Input: part model. Units: mm. Frame: model coordinates. Face numbers are marked on the shaded views. A direction names the side the tool comes from. Give positions to 0.01 mm unless a question says otherwise; leave off trailing zeros. Write each loop counter-clockwise with the first axis right and the second up, starting at its lowest first coordinate (ties: lowest second). Pieces come first, ordered by that corner, then holes. Notation, with made-up numbers: (53.25, 43.5) - (73.25, 43.5) arc R21 ccw to (73.25, 55.5) - close; hole circle Ø10 at (48, 78). An arc over 180 degrees is marked (long way). Answer as CSV lines item,"result".
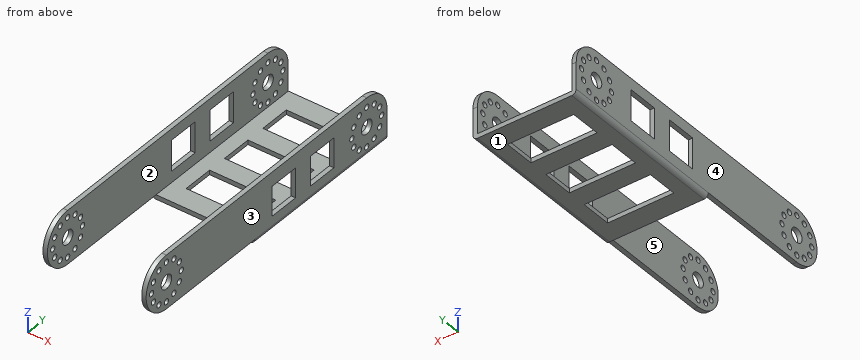
```python
from build123d import *

# Parameters (mm, degrees)
ESQUISSE2_W        = 33.6
ESQUISSE2_H        = 62
ESQUISSE2_W_2      = 23.6
ESQUISSE2_H_2      = 11
BOSS_EXTRU_1_DEPTH = 1.5875
ESQUISSE3_R        = 2.5
ESQUISSE3_R_2      = 1
ESQUISSE3_W        = 10.5875
ESQUISSE3_H        = 11
BOSS_EXTRU_2_DEPTH = 1.5875
CONG_3_R           = 1.5875
CONG_4_R           = 9.5
ESQUISSE4_R        = 2.5
ESQUISSE4_R_2      = 1
ESQUISSE4_W        = 11.003569346
ESQUISSE4_H        = 11
BOSS_EXTRU_3_DEPTH = 1.5875
CONG_6_R           = 1.5875
CONG_7_R           = 9.5


with BuildPart() as part:
    # Esquisse2 → Boss.-Extru.1 (new body)
    with BuildSketch(Plane.XY):
        Rectangle(ESQUISSE2_W, ESQUISSE2_H)
        Rectangle(ESQUISSE2_W_2, ESQUISSE2_H_2, mode=Mode.SUBTRACT)
        with Locations((0, 18)):
            Rectangle(ESQUISSE2_W_2, ESQUISSE2_H_2, mode=Mode.SUBTRACT)
        with Locations((0, -18)):
            Rectangle(ESQUISSE2_W_2, ESQUISSE2_H_2, mode=Mode.SUBTRACT)
    extrude(amount=BOSS_EXTRU_1_DEPTH)


with BuildPart() as body_2:
    # Esquisse3 → Boss.-Extru.2 (new body)
    with BuildSketch(Plane(origin=(16.8, 0, 0), x_dir=(0, 0, -1), z_dir=(1, 0, 0))):
        with BuildLine():
            Line((-20.5875, 31), (0, 31))
            Line((0, 31), (0, -31))
            Line((0, -31), (-1.5875, -31))
            Line((-1.5875, -31), (-1.5875, -72.5))
            ThreePointArc((-1.5875, -72.5), (-11.0875, -82), (-20.5875, -72.5))
            Line((-20.5875, -72.5), (-20.5875, -31))
            Line((-20.5875, -31), (-20.5875, 31))
        make_face()
        with Locations((-11.0875, -72.5)):
            Circle(ESQUISSE3_R, mode=Mode.SUBTRACT)
        with Locations((-11.0875, -79.5)):
            Circle(ESQUISSE3_R_2, mode=Mode.SUBTRACT)
        with Locations((-14.5875, -78.562177826)):
            Circle(ESQUISSE3_R_2, mode=Mode.SUBTRACT)
        with Locations((-17.149677826, -76)):
            Circle(ESQUISSE3_R_2, mode=Mode.SUBTRACT)
        with Locations((-18.0875, -72.5)):
            Circle(ESQUISSE3_R_2, mode=Mode.SUBTRACT)
        with Locations((-17.149677826, -69)):
            Circle(ESQUISSE3_R_2, mode=Mode.SUBTRACT)
        with Locations((-14.5875, -66.437822174)):
            Circle(ESQUISSE3_R_2, mode=Mode.SUBTRACT)
        with Locations((-11.0875, -65.5)):
            Circle(ESQUISSE3_R_2, mode=Mode.SUBTRACT)
        with Locations((-7.5875, -66.437822174)):
            Circle(ESQUISSE3_R_2, mode=Mode.SUBTRACT)
        with Locations((-5.025322174, -69)):
            Circle(ESQUISSE3_R_2, mode=Mode.SUBTRACT)
        with Locations((-4.0875, -72.5)):
            Circle(ESQUISSE3_R_2, mode=Mode.SUBTRACT)
        with Locations((-5.025322174, -76)):
            Circle(ESQUISSE3_R_2, mode=Mode.SUBTRACT)
        with Locations((-7.5875, -78.562177826)):
            Circle(ESQUISSE3_R_2, mode=Mode.SUBTRACT)
        with Locations((-10.29375, 21.5)):
            Circle(ESQUISSE3_R, mode=Mode.SUBTRACT)
        with Locations((-10.29375, 28.5)):
            Circle(ESQUISSE3_R_2, mode=Mode.SUBTRACT)
        with Locations((-6.79375, 27.562177826)):
            Circle(ESQUISSE3_R_2, mode=Mode.SUBTRACT)
        with Locations((-4.231572174, 25)):
            Circle(ESQUISSE3_R_2, mode=Mode.SUBTRACT)
        with Locations((-3.29375, 21.5)):
            Circle(ESQUISSE3_R_2, mode=Mode.SUBTRACT)
        with Locations((-4.231572174, 18)):
            Circle(ESQUISSE3_R_2, mode=Mode.SUBTRACT)
        with Locations((-6.79375, 15.437822174)):
            Circle(ESQUISSE3_R_2, mode=Mode.SUBTRACT)
        with Locations((-10.29375, 14.5)):
            Circle(ESQUISSE3_R_2, mode=Mode.SUBTRACT)
        with Locations((-13.79375, 15.437822174)):
            Circle(ESQUISSE3_R_2, mode=Mode.SUBTRACT)
        with Locations((-16.355927826, 18)):
            Circle(ESQUISSE3_R_2, mode=Mode.SUBTRACT)
        with Locations((-17.29375, 21.5)):
            Circle(ESQUISSE3_R_2, mode=Mode.SUBTRACT)
        with Locations((-16.355927826, 25)):
            Circle(ESQUISSE3_R_2, mode=Mode.SUBTRACT)
        with Locations((-13.79375, 27.562177826)):
            Circle(ESQUISSE3_R_2, mode=Mode.SUBTRACT)
        with Locations((-10.29375, 0.597470968)):
            Rectangle(ESQUISSE3_W, ESQUISSE3_H, mode=Mode.SUBTRACT)
        with Locations((-10.29375, -17.402529032)):
            Rectangle(ESQUISSE3_W, ESQUISSE3_H, mode=Mode.SUBTRACT)
    extrude(amount=BOSS_EXTRU_2_DEPTH)

    # Congé3
    cong_3_edges = [body_2.edges().sort_by_distance(p)[0] for p in [
        (18.3875, 0, 0),
    ]]
    fillet(cong_3_edges, radius=CONG_3_R - 0.0001)  # a hair under: the kernel refuses the full size

    # Congé4
    cong_4_edges = [body_2.edges().sort_by_distance(p)[0] for p in [
        (17.59375, 31, 20.5875),
    ]]
    fillet(cong_4_edges, radius=CONG_4_R)

    # Intersect1: read off the stored shape, not the designer's step
    # Intersect1: union part
    add(part.part)

    # Esquisse4 → Boss.-Extru.3 (add)
    with BuildSketch(Plane.ZY.offset(16.8)):
        with BuildLine():
            Line((1.5875, 31), (0, 31))
            Line((0, 31), (0, -31))
            Line((0, -31), (1.5875, -31))
            Line((1.5875, -31), (1.5875, -72.5))
            ThreePointArc((1.5875, -72.5), (11.0875, -82), (20.5875, -72.5))
            Line((20.5875, -72.5), (20.5875, 31))
            Line((20.5875, 31), (1.5875, 31))
        make_face()
        with Locations(Location((11.0875, -72.5, 0), (0, 0, 180))):
            Circle(ESQUISSE4_R, mode=Mode.SUBTRACT)
        with Locations(Location((11.0875, -79.5, 0), (0, 0, 180))):
            Circle(ESQUISSE4_R_2, mode=Mode.SUBTRACT)
        with Locations(Location((7.5875, -78.562177826, 0), (0, 0, 180))):
            Circle(ESQUISSE4_R_2, mode=Mode.SUBTRACT)
        with Locations(Location((5.025322174, -76, 0), (0, 0, 180))):
            Circle(ESQUISSE4_R_2, mode=Mode.SUBTRACT)
        with Locations(Location((4.0875, -72.5, 0), (0, 0, 180))):
            Circle(ESQUISSE4_R_2, mode=Mode.SUBTRACT)
        with Locations(Location((5.025322174, -69, 0), (0, 0, 180))):
            Circle(ESQUISSE4_R_2, mode=Mode.SUBTRACT)
        with Locations(Location((7.5875, -66.437822174, 0), (0, 0, 180))):
            Circle(ESQUISSE4_R_2, mode=Mode.SUBTRACT)
        with Locations(Location((11.0875, -65.5, 0), (0, 0, 180))):
            Circle(ESQUISSE4_R_2, mode=Mode.SUBTRACT)
        with Locations(Location((14.5875, -66.437822174, 0), (0, 0, 180))):
            Circle(ESQUISSE4_R_2, mode=Mode.SUBTRACT)
        with Locations(Location((17.149677826, -69, 0), (0, 0, 180))):
            Circle(ESQUISSE4_R_2, mode=Mode.SUBTRACT)
        with Locations(Location((18.0875, -72.5, 0), (0, 0, 180))):
            Circle(ESQUISSE4_R_2, mode=Mode.SUBTRACT)
        with Locations(Location((17.149677826, -76, 0), (0, 0, 180))):
            Circle(ESQUISSE4_R_2, mode=Mode.SUBTRACT)
        with Locations(Location((14.5875, -78.562177826, 0), (0, 0, 180))):
            Circle(ESQUISSE4_R_2, mode=Mode.SUBTRACT)
        with Locations(Location((10.29375, 21.5, 0), (0, 0, 180))):
            Circle(ESQUISSE4_R, mode=Mode.SUBTRACT)
        with Locations(Location((6.79375, 15.437822174, 0), (0, 0, 180))):
            Circle(ESQUISSE4_R_2, mode=Mode.SUBTRACT)
        with Locations(Location((4.231572174, 18, 0), (0, 0, 180))):
            Circle(ESQUISSE4_R_2, mode=Mode.SUBTRACT)
        with Locations(Location((10.29375, 14.5, 0), (0, 0, 180))):
            Circle(ESQUISSE4_R_2, mode=Mode.SUBTRACT)
        with Locations(Location((3.29375, 21.5, 0), (0, 0, 180))):
            Circle(ESQUISSE4_R_2, mode=Mode.SUBTRACT)
        with Locations(Location((4.231572174, 25, 0), (0, 0, 180))):
            Circle(ESQUISSE4_R_2, mode=Mode.SUBTRACT)
        with Locations(Location((6.79375, 27.562177826, 0), (0, 0, 180))):
            Circle(ESQUISSE4_R_2, mode=Mode.SUBTRACT)
        with Locations(Location((10.29375, 28.5, 0), (0, 0, 180))):
            Circle(ESQUISSE4_R_2, mode=Mode.SUBTRACT)
        with Locations(Location((13.79375, 27.562177826, 0), (0, 0, 180))):
            Circle(ESQUISSE4_R_2, mode=Mode.SUBTRACT)
        with Locations(Location((16.355927826, 25, 0), (0, 0, 180))):
            Circle(ESQUISSE4_R_2, mode=Mode.SUBTRACT)
        with Locations(Location((17.29375, 21.5, 0), (0, 0, 180))):
            Circle(ESQUISSE4_R_2, mode=Mode.SUBTRACT)
        with Locations(Location((16.355927826, 18, 0), (0, 0, 180))):
            Circle(ESQUISSE4_R_2, mode=Mode.SUBTRACT)
        with Locations(Location((13.79375, 15.437822174, 0), (0, 0, 180))):
            Circle(ESQUISSE4_R_2, mode=Mode.SUBTRACT)
        with Locations((11.085715327, -0.168943848)):
            Rectangle(ESQUISSE4_W, ESQUISSE4_H, mode=Mode.SUBTRACT)
        with Locations((11.085715327, -18.168943848)):
            Rectangle(ESQUISSE4_W, ESQUISSE4_H, mode=Mode.SUBTRACT)
    extrude(amount=BOSS_EXTRU_3_DEPTH)

    # Congé6
    cong_6_edges = [body_2.edges().sort_by_distance(p)[0] for p in [
        (-18.3875, 0, 0),
    ]]
    fillet(cong_6_edges, radius=CONG_6_R)

    # Congé7
    cong_7_edges = [body_2.edges().sort_by_distance(p)[0] for p in [
        (-17.59375, 31, 20.5875),
    ]]
    fillet(cong_7_edges, radius=CONG_7_R)


solid = body_2.part
```
Item 1: Reachability of the marked faces 1 and 2 from +Z, -Z, +X, -X, +Y, -Y: full face, straight path, thin tool, end or side. Return the list, or none.
The answers:
face 1,"-Z, +X, -X, +Y, -Y"
face 2,"+Z, +Y, -Y"
Item 2: Cut plane C-C on y = 0. Return the cut outline in (x, z) (1 decimal).
The answers:
outline,"(-18.4, 1.6) arc R1.6 ccw to (-16.8, 0) - (-11.8, 0) - (-11.8, 1.6) - (-16.8, 1.6) - (-16.8, 5.6) - (-18.4, 5.6) - close; (-18.4, 16.6) - (-16.8, 16.6) - (-16.8, 20.6) - (-18.4, 20.6) - close; (11.8, 0) - (16.8, 0) arc R1.6 ccw to (18.4, 1.6) - (18.4, 5) - (16.8, 5) - (16.8, 1.6) - (11.8, 1.6) - close; (16.8, 15.6) - (18.4, 15.6) - (18.4, 20.6) - (16.8, 20.6) - close"
Item 3: Cut plane B-B on x = 2. Return the cut outline in (y, z).
The answers:
outline,"(-31, 0) - (-23.5, 0) - (-23.5, 1.59) - (-31, 1.59) - close; (-12.5, 0) - (-5.5, 0) - (-5.5, 1.59) - (-12.5, 1.59) - close; (5.5, 0) - (12.5, 0) - (12.5, 1.59) - (5.5, 1.59) - close; (23.5, 0) - (31, 0) - (31, 1.59) - (23.5, 1.59) - close"
Item 4: Cut plane A-A on y = -69. Return the cut outline in (x, z), plus the area to 3 significant figures.
The answers:
outline,"(-18.39, 1.59) - (-16.8, 1.59) - (-16.8, 4.03) - (-18.39, 4.03) - close; (-18.39, 6.03) - (-16.8, 6.03) - (-16.8, 16.15) - (-18.39, 16.15) - close; (-18.39, 18.15) - (-16.8, 18.15) - (-16.8, 20.59) - (-18.39, 20.59) - close; (16.8, 1.59) - (18.39, 1.59) - (18.39, 4.03) - (16.8, 4.03) - close; (16.8, 6.03) - (18.39, 6.03) - (18.39, 16.15) - (16.8, 16.15) - close; (16.8, 18.15) - (18.39, 18.15) - (18.39, 20.59) - (16.8, 20.59) - close"
area,"47.6 mm²"
Item 5: Ray query, line 1 (Z direction, x = -17.35, y = -72.5); line 2 (X direction, y = -58, z = 11); line 3 (Z direction, x = 17, y = -72). Return the intervals inside material, ascending. Write a range as from..to.
The answers:
line 1,"1.59..3.09, 5.09..8.59, 13.59..17.09, 19.09..20.59"
line 2,"-18.39..-16.8, 16.8..18.39"
line 3,"1.59..3.22, 4.95..8.64, 13.54..17.22, 18.95..20.59"
Item 6: Cut plane D-D on y = 25. Return the cut outline in (x, z) (1 decimal).
The answers:
outline,"(-18.4, 1.6) arc R1.6 ccw to (-16.8, 0) - (16.8, 0) arc R1.6 ccw to (18.4, 1.6) - (18.4, 3.2) - (16.8, 3.2) - (16.8, 1.6) - (-16.8, 1.6) - (-16.8, 3.2) - (-18.4, 3.2) - close; (-18.4, 5.2) - (-16.8, 5.2) - (-16.8, 15.4) - (-18.4, 15.4) - close; (-18.4, 17.4) - (-16.8, 17.4) - (-16.8, 19.9) - (-18.4, 19.9) - close; (16.8, 5.2) - (18.4, 5.2) - (18.4, 15.4) - (16.8, 15.4) - close; (16.8, 17.4) - (18.4, 17.4) - (18.4, 19.9) - (16.8, 19.9) - close"
Item 7: Mould query, pull axis X, two halves, no side actions, for the marked faces 3, 4 and 5. Classes: +X half, -X half, draft (parallel to the pull), parting line (faces both ways), or undercut.
The answers:
face 3,"+X half"
face 4,"-X half"
face 5,"undercut"
Item 8: Contact query for flat-ended pins moving along their axis: pin 1 (0.8 mm diameter, centred on y = 16, z = 1, fed in from +X); pin 2 (8 mm diameter, centred on x = -14.5, z = 18.5, fed in from +Y); pin 3 (1.7 mm diameter, centred on x = -4, z = 1, fed in from -Y). Output: stop coordinate, or through.
The answers:
pin 1,"x = 18.38"
pin 2,"y = 30.05"
pin 3,"y = -31"
